Work out the finished part from the listing and answer in its coordinate system (mm). A direction names the side the tool comes from. Coordinates: 2 decimals unless noted, no trailing zeros. Write each loop counter-clockwise with the first axis right and the second up, starting at its lowest first coordinate (ties: lowest second). Pieces come first, ordered by that corner, then holes. Notation, with made-up numbers: (-24, 75.25) - (-13, 75.25) arc R22 ccw to (-13, 89.25) - close; hole circle Ø1 at (32, 63). An arc over 180 degrees is marked (long way). Use one line per item in the form item = value. Start each with the question number.
Item 1: A cutting plane is placed at C-C (z = -4.75). Write down the section's boundary in (x, y).
Item 2: Determine the mould class of faces 4 (the flat face through (10, 1, -7)), 5 (the flat face through (7, -10, -7)), 6 (the flat face through (5, 2, -7)), 7 (the cylindrical face through (6.763, 3.676, -7.521)) for opening direction X: released by +X, released by -X, zero draft, split by the parting line, or undercut.
Item 3: Consider probe 1 along Y at (x, z) = (7.5, -7.35); probe 2 along Y at (x, z) = (1, -4.5); probe 3 along Z at (x, y) = (9.25, 1.5). Determine where each line is inside the solid, lowest interval first.
Item 4: Given pin 1 (6 mm diameter, centred on y = 3.5, z = -5, fed in from -X); pin 2 (2.5 mm diameter, centred on x = 7.5, y = 3, fed in from +Z); pin 3 (2.5 mm diameter, centred on y = 1.5, z = -7.5, fed in from +X), each flat-ended and moving along its own axis, determine where each tip first touches the part or whether it passes through.
Item 5: A cutting plane is placed at B-B (x = 11.25). Write down the section's boundary in (y, z), then the cut area to 3 significant figures.
Item 6: A cutting plane is placed at A-A (x = 7.5). Write down the section's boundary in (y, z).
Item 7: For faces 1 (the flat face through (7.5, 1.6, -9)), 2 (the flat face through (7.5, 1.6, -6)), 3 (the flat face through (0, -5, -8)), determine the directions among +Z, -Z, +X, -X, +Y, -Y from which every point of the face is accessible in a straight line to the end or side of a thin tool.
from build123d import *

# Parameters (mm, degrees)
SKETCH1_W           = 15
SKETCH1_H           = 15
BOSS_EXTRUDE1_DEPTH = 10
SKETCH4_R           = 1
BOSS_EXTRUDE2_DEPTH = 1.5


with BuildPart() as part:
    # Sketch1 → Boss-Extrude1 (new body)
    with BuildSketch(Plane.XZ):
        with Locations((7.5, -7.5)):
            Rectangle(SKETCH1_W, SKETCH1_H)
    extrude(amount=BOSS_EXTRUDE1_DEPTH)

    # Sketch4 → Boss-Extrude2 (add, symmetric)
    with BuildSketch(Plane.XY.offset(-7.5)):
        with BuildLine():
            ThreePointArc((10, 3), (7.5, 5.5), (5, 3))
            Line((5, 3), (5, 0))
            Line((5, 0), (10, 0))
            Line((10, 0), (10, 3))
        make_face()
        with Locations((7.5, 3)):
            Circle(SKETCH4_R, mode=Mode.SUBTRACT)
    extrude(amount=BOSS_EXTRUDE2_DEPTH, both=True)


solid = part.part
Answer:
q1.outline = (0, -10) - (15, -10) - (15, 0) - (0, 0) - close
q2.face_4 = released by +X
q2.face_5 = zero draft
q2.face_6 = released by -X
q2.face_7 = undercut
q3.probe_1 = -10 to 2, 4 to 5.5
q3.probe_2 = -10 to 0
q3.probe_3 = -9 to -6
q4.pin_1 = 5
q4.pin_2 = -6
q4.pin_3 = 10
q5.outline = (-10, -15) - (0, -15) - (0, 0) - (-10, 0) - close
q5.area = 150 mm²
q6.outline = (-10, -15) - (0, -15) - (0, -9) - (2, -9) - (2, -6) - (0, -6) - (0, 0) - (-10, 0) - close; (4, -9) - (5.5, -9) - (5.5, -6) - (4, -6) - close
q7.face_1 = -Z, +X, -X, +Y
q7.face_2 = +Z, +X, -X, +Y
q7.face_3 = +Z, -Z, -X, +Y, -Y
